Part model, mm, in its own coordinate system. Face numbers are marked on the shaded views. A direction names the side the tool comes from. Coordinates: 2 decimals unless noted, no trailing zeros. Loops run counter-clockwise (first coordinate to the right, second up) from the corner with the lowest first, then second, coordinate; pieces in that order, holes last. Notation, with made-up numbers: (-18.5, 41) - (8.5, 41) arc R20 cw to (8.5, 65) - close; hole circle Ø1 at (24.5, 30.25). An arc over 180 degrees is marked (long way). Answer as CSV lines item,"result".
from build123d import *

# Parameters (mm, degrees)
SKETCH1_W                      = 83
SKETCH1_H                      = 105
SKETCH1_R                      = 1.75
BOSS_EXTRUDE1_DEPTH            = 8
CBORE_FOR_M3_SHCS1_OUTLINE_R   = 3.25
CBORE_FOR_M3_SHCS1_DEPTH       = 3
CBORE_START                    = 3
CBORE_FOR_M3_SHCS1_2_OUTLINE_R = 1.8
CBORE_FOR_M3_SHCS1_2_DEPTH     = 5
CUT_EXTRUDE1_DEPTH             = 4
SKETCH6_W                      = 5
SKETCH6_H                      = 20
BOSS_EXTRUDE2_DEPTH            = 8.8
SKETCH7_W                      = 3.2
SKETCH7_H                      = 6.8
CUT_EXTRUDE2_DEPTH             = 103.793190436
FILLET1_SIZE                   = 6
FILLET1_SIZE_2                 = 8
FILLET2_R                      = 1
SKETCH8_W                      = 67
SKETCH8_H                      = 93
BOSS_EXTRUDE4_DEPTH            = 15
CUT_EXTRUDE3_DEPTH             = 90
SKETCH12_W                     = 64.6
SKETCH12_H                     = 1.5
CUT_EXTRUDE4_DEPTH             = 1


# Read off the part's stored shape, not the designer's step: CBORE for M3 SHCS1
with BuildPart() as part:
    # Sketch1 → Boss-Extrude1 (new body)
    with BuildSketch(Plane(origin=(0, 0, 0), x_dir=(1, 0, 0), z_dir=(0, 1, 0))):
        with Locations((41.5, 52.5)):
            Rectangle(SKETCH1_W, SKETCH1_H)
        with Locations(Location((5, 25, 0), (0, 0, 270))):
            Circle(SKETCH1_R, mode=Mode.SUBTRACT)
        with Locations(Location((78, 25, 0), (0, 0, 90))):
            Circle(SKETCH1_R, mode=Mode.SUBTRACT)
    extrude(amount=BOSS_EXTRUDE1_DEPTH)

    # CBORE for M3 SHCS1 outline → CBORE for M3 SHCS1 (cut)
    with BuildSketch(Plane(origin=(0, 0, 0), x_dir=(1, 0, 0), z_dir=(0, 1, 0))):
        with Locations((14.475, 93.775)):
            Circle(CBORE_FOR_M3_SHCS1_OUTLINE_R)
        with Locations((68.525, 93.775)):
            Circle(CBORE_FOR_M3_SHCS1_OUTLINE_R)
        with Locations((68.525, 11.225)):
            Circle(CBORE_FOR_M3_SHCS1_OUTLINE_R)
        with Locations((14.475, 11.225)):
            Circle(CBORE_FOR_M3_SHCS1_OUTLINE_R)
    extrude(amount=CBORE_FOR_M3_SHCS1_DEPTH, mode=Mode.SUBTRACT)

    # CBORE for M3 SHCS1 2 outline → CBORE for M3 SHCS1 2 (cut)
    with BuildSketch(Plane(origin=(0, 0, 0), x_dir=(1, 0, 0), z_dir=(0, 1, 0)).offset(CBORE_START)):
        with Locations((14.475, 93.775)):
            Circle(CBORE_FOR_M3_SHCS1_2_OUTLINE_R)
        with Locations((68.525, 93.775)):
            Circle(CBORE_FOR_M3_SHCS1_2_OUTLINE_R)
        with Locations((68.525, 11.225)):
            Circle(CBORE_FOR_M3_SHCS1_2_OUTLINE_R)
        with Locations((14.475, 11.225)):
            Circle(CBORE_FOR_M3_SHCS1_2_OUTLINE_R)
    extrude(amount=CBORE_FOR_M3_SHCS1_2_DEPTH, mode=Mode.SUBTRACT)

    # Sketch5 → Cut-Extrude1 (cut)
    with BuildSketch(Plane(origin=(0, 8, 0), x_dir=(1, 0, 0), z_dir=(0, 1, 0))):
        with BuildLine():
            Line((19.475, 93.775), (63.525, 93.775))
            ThreePointArc((63.525, 93.775), (64.989466094, 90.239466094), (68.525, 88.775))
            Line((68.525, 88.775), (68.525, 16.225))
            ThreePointArc((68.525, 16.225), (64.989466094, 14.760533906), (63.525, 11.225))
            Line((63.525, 11.225), (19.475, 11.225))
            ThreePointArc((19.475, 11.225), (18.010533906, 14.760533906), (14.475, 16.225))
            Line((14.475, 16.225), (14.475, 88.775))
            ThreePointArc((14.475, 88.775), (18.010533906, 90.239466094), (19.475, 93.775))
        make_face()
    extrude(amount=-CUT_EXTRUDE1_DEPTH, mode=Mode.SUBTRACT)

    # Sketch6 → Boss-Extrude2 (add)
    with BuildSketch(Plane.XZ):
        with Locations((13.975, -50)):
            Rectangle(SKETCH6_W, SKETCH6_H)
    extrude(amount=BOSS_EXTRUDE2_DEPTH)

    # Sketch7 → Cut-Extrude2 (cut, through all)
    with BuildSketch(Plane(origin=(0, 0, -60), x_dir=(-1, 0, 0), z_dir=(0, 0, -1))):
        with Locations((-13.075, -3.4)):
            Rectangle(SKETCH7_W, SKETCH7_H)
    extrude(amount=-CUT_EXTRUDE2_DEPTH, mode=Mode.SUBTRACT)

    # Fillet1
    # an asymmetric fillet: 8, 6 mm, written as the material it adds along each edge
    with BuildSketch(Plane(origin=(16.475, 0, -40), x_dir=(1, 0, 0), z_dir=(0, 0, -1))) as fillet1_piece_1:
        with BuildLine():
            Bezier((FILLET1_SIZE, 0), (0, 0), (0, FILLET1_SIZE_2), weights=[1, 0.707106781, 1])
            Line((0, FILLET1_SIZE_2), (0, 0))
            Line((0, 0), (FILLET1_SIZE, 0))
        make_face()
    extrude(amount=20)

    # Fillet2
    fillet2_edges = [part.edges().sort_by_distance(p)[0] for p in [
        (83, 8, -52.5),
        (41.5, 8, -105),
        (0, 8, -52.5),
        (41.5, 0, 0),
        (0, 0, -52.5),
        (0, 4, -105),
        (83, 4, -105),
        (83, 4, 0),
        (0, 4, 0),
        (41.5, 8, 0),
    ]]
    fillet(fillet2_edges, radius=FILLET2_R)

    # Sketch8 → Boss-Extrude4 (add)
    with BuildSketch(Plane(origin=(0, 8, 0), x_dir=(1, 0, 0), z_dir=(0, 1, 0))):
        with Locations((41.5, 47.5)):
            Rectangle(SKETCH8_W, SKETCH8_H)
    extrude(amount=BOSS_EXTRUDE4_DEPTH)

    # Sketch11 → Cut-Extrude3 (cut)
    with BuildSketch(Plane(origin=(0, 0, -94), x_dir=(-1, 0, 0), z_dir=(0, 0, -1))):
        Polygon((-72.5, 8), (-10.5, 8), (-10.5, 19.5), (-9.2, 19.5), (-9.2, 21), (-10.5, 21), (-10.5, 23), (-72.5, 23), (-72.5, 21), (-73.8, 21), (-73.8, 19.5), (-72.5, 19.5), align=None)
    extrude(amount=-CUT_EXTRUDE3_DEPTH, mode=Mode.SUBTRACT)

    # Sketch12 → Cut-Extrude4 (cut)
    with BuildSketch(Plane(origin=(0, 0, -4), x_dir=(-1, 0, 0), z_dir=(0, 0, -1))):
        with Locations((-41.5, 20.25)):
            Rectangle(SKETCH12_W, SKETCH12_H)
    extrude(amount=-CUT_EXTRUDE4_DEPTH, mode=Mode.SUBTRACT)


solid = part.part
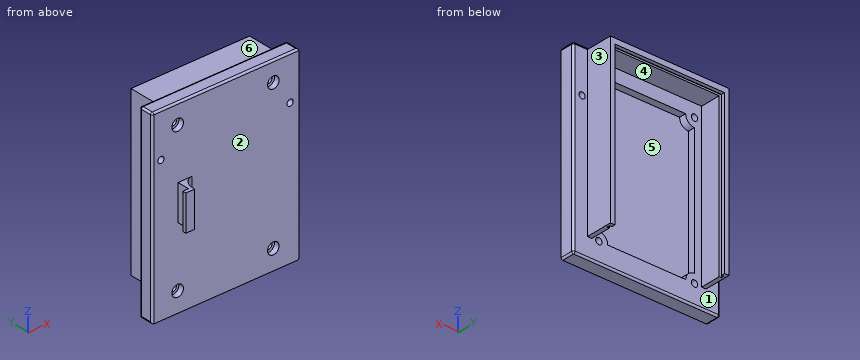
Q1. Which spindle directions (+Z, -Z, +X, -X, +Y, -Y) get a long thin tool onto all of the face, cutting with end or side? Do the marked faces 4, 5 and 6. Say none if no direction does.
Results:
face 4,"-Z, +Y"
face 5,"+Y"
face 6,"+Z, +X, -X, +Y"
Q2. Saw through at C-C (x = 57.5). Give the cut face in (y, z) (3 decimals), then the cut area to 3 significant figures.
Results:
outline,"(0, -105) - (7, -105) arc R1 ccw to (8, -104) - (8, -93.775) - (4, -93.775) - (4, -11.225) - (8, -11.225) - (8, -4) - (19.5, -4) - (19.5, -3) - (21, -3) - (21, -4) - (23, -4) - (23, -1) - (8, -1) arc R1 ccw to (7, 0) - (1, 0) arc R1 ccw to (0, -1) - close"
area,"553 mm^2"
Q3. Saw through at B-B (x = 78). Give the cut face in (y, z), then the cut area to 3 significant figures.
Results:
outline,"(0, -105) - (7, -105) arc R1 ccw to (8, -104) - (8, -26.75) - (0, -26.75) - close; (0, -23.25) - (8, -23.25) - (8, -1) arc R1 ccw to (7, 0) - (1, 0) arc R1 ccw to (0, -1) - close"
area,"811 mm^2"
Q4. Two-plate mould, pull along X, no slides. Class the marked faces 1, 2 and 3: released by +X, released by -X, zero draft, split by the parting line, or undercut.
Results:
face 1,"undercut"
face 2,"zero draft"
face 3,"released by +X"
Q5. Wall check: L1, parallel to X at y = 18, z = -41.5; L2, parallel to Z at x = 62, y = 7 (3 decimals); L3, parallel to X at y = 5, z = -90. Give the ranges that are in metal, low to high.
Results:
L1,"x = 8 to 10.5, 72.5 to 75"
L2,"z = -105 to -93.775, -11.225 to 0"
L3,"x = 0 to 17.75, 65.25 to 83"
Q6. Flat gauge pins, fed straight in: pin 1 (7 mm diameter, centred on x = 69, z = -10, fed in from -Y); pin 2 (1.5 mm diameter, centred on x = 42, y = 10, fed in from -Z); pin 3 (3 mm diameter, centred on x = 68.525, z = -93.775, fed in from -Y); pin 4 (1.2 mm diameter, centred on y = 20, z = -41, fed in from -X). Where does each tip first touch, or does it go through?
Results:
pin 1,"stops at y = 0"
pin 2,"stops at z = -4"
pin 3,"passes through"
pin 4,"stops at x = 8"
Q7. Saw through at D-D (z = -21). Give the cut face in (x, y) (3 decimals).
Results:
outline,"(0, 1) arc R1 ccw to (1, 0) - (83, 0) - (83, 7) arc R1 ccw to (82, 8) - (75, 8) - (75, 23) - (72.5, 23) - (72.5, 21) - (73.8, 21) - (73.8, 19.5) - (72.5, 19.5) - (72.5, 8) - (68.525, 8) - (68.525, 4) - (14.475, 4) - (14.475, 8) - (10.5, 8) - (10.5, 19.5) - (9.2, 19.5) - (9.2, 21) - (10.5, 21) - (10.5, 23) - (8, 23) - (8, 8) - (1, 8) arc R1 ccw to (0, 7) - close"
Q8. Saw through at A-A (y = 11). Give the cut face in (x, z), then the cut area to 3 significant figures.
Results:
outline,"(8, -94) - (10.5, -94) - (10.5, -4) - (72.5, -4) - (72.5, -94) - (75, -94) - (75, -1) - (8, -1) - close"
area,"651 mm^2"
